Source: CAD feature listing. Evaluate the final solid. Frame: model axes, mm. Face numbers are marked on the shaded views. A direction names the side the tool comes from. Give positions to 0.01 mm unless a question says otherwise; leave off trailing zeros. Write each loop counter-clockwise with the first axis right and the second up, starting at its lowest first coordinate (ties: lowest second). Pieces come first, ordered by that corner, then holes. Notation, with made-up numbers: M 46.25,34.5 L 87.25,34.5 A25 ccw 87.25,58.5 Z; hole C -7.75,-1 d11. An arc over 180 degrees is marked long. Answer as a JSON object with one key per item and string values. Group by question number.
```python
from build123d import *

# Parameters (mm, degrees)
F0_W     = 177.8
F0_H     = 152.4
F1_DEPTH = 81.59288
F2_R     = 63.5
F3_DEPTH = 51.22014
F4_R     = 5.08
F5_R     = 5.08
F6_T     = -2.54


with BuildPart() as f1:
    # F0 (on Front) → F1 (new body)
    with BuildSketch(Plane.XZ):
        Rectangle(F0_W, F0_H)
    extrude(amount=-F1_DEPTH)

    # F2 (on face) → F3 (join)
    with BuildSketch(Plane(origin=(0, 81.59288, 0), x_dir=(-1, 0, 0), z_dir=(0, 1, 0))):
        Circle(F2_R)
    extrude(amount=F3_DEPTH)

    # F4
    f4_edges = [f1.edges().sort_by_distance(p)[0] for p in [
        (63.5, 81.59288, 0),
        (63.5, 132.81302, 0),
        (-88.9, 40.79644, 76.2),
        (88.9, 40.79644, 76.2),
        (-88.9, 40.79644, -76.2),
        (88.9, 40.79644, -76.2),
    ]]
    fillet(f4_edges, radius=F4_R)

    # F5
    f5_edges = [f1.edges().sort_by_distance(p)[0] for p in [
        (0, 81.59288, -76.2),
    ]]
    fillet(f5_edges, radius=F5_R)

    # F6
    f6_openings = [f1.faces().sort_by_distance(p)[0] for p in [
        (0, 0, 0),
    ]]
    offset(amount=F6_T, openings=f6_openings)


solid = f1.part
```
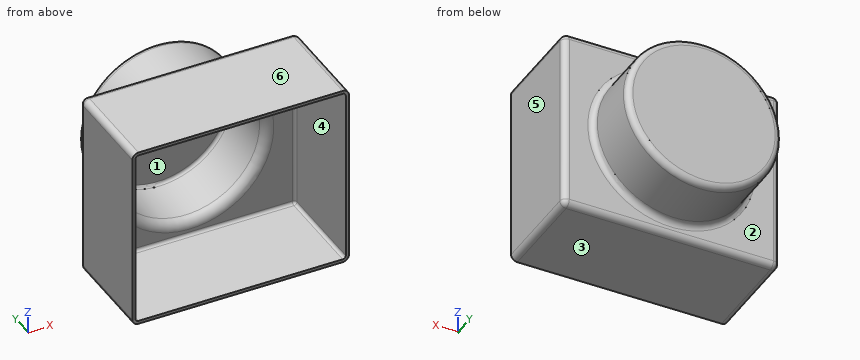
(1) Pull-direction query (Z, two-part tool) for the marked faces 4, 5 and 6; classes: pulls with the +Z half, pulls with the -Z half, needs draft (parallel to the pull), parting line crosses it, or undercut.
(2) Contact query for flat-ended pins moving along their axis: pin 1 Ø6 at (y, z) = (111, 50.5) entering from -X; pin 2 Ø2 at (x, y) = (28, 79.5) entering from +Z; pin 3 Ø6 at (y, z) = (81.5, 29) entering from +X. Output: stop coordinate, or through.
(3) Section A-A, the plane y = 12.5. Return loops of the section in (x, z).
(4) Access query for the marked faces 1, 2 and 3. Directions: +Z, -Z, +X, -X, +Y, -Y. A direction counts if a zero-diameter tool reaches every point of the face in a straight line with its end or side. Return the directions, or none.
(5) Section B-B, the plane x = 0. Return loops of the section in (y, z), plus the area to 3 significant figures.
(6) Section C-C, the plane z = 0. Return loops of the section in (x, y), plus the area to 3 significant figures.
(7) Ray query, L1, parallel to X at y = 63, z = 43.5; L2, parallel to Z at x = 0, y = 117; L3, parallel to X at y = 126, z = -2. Return the intervals inside material, ascending. Write a range as [from, to].
Reported:
{
 "1": {"face 4": "undercut", "face 5": "needs draft", "face 6": "pulls with the +Z half"},
 "2": {"pin 1": "stops at x = -42.14", "pin 2": "stops at z = 75.8", "pin 3": "stops at x = 88.5"},
 "3": {"outline": "M -88.9,-71.12 A5.08 ccw -83.82,-76.2 L 83.82,-76.2 A5.08 ccw 88.9,-71.12 L 88.9,71.12 A5.08 ccw 83.82,76.2 L -83.82,76.2 A5.08 ccw -88.9,71.12 Z; hole M -86.36,-71.12 A2.54 ccw -83.82,-73.66 L 83.82,-73.66 A2.54 ccw 86.36,-71.12 L 86.36,71.12 A2.54 ccw 83.82,73.66 L -83.82,73.66 A2.54 ccw -86.36,71.12 Z"},
 "4": {"face 1": "-Y", "face 2": "+Y", "face 3": "-Z, +X, -X, +Y, -Y"},
 "5": {"outline": "M 0,-76.2 L 76.51,-76.2 A5.08 ccw 81.59,-71.12 L 81.59,-68.58 A5.08 cw 86.67,-63.5 L 127.73,-63.5 A5.08 ccw 132.81,-58.42 L 132.81,58.42 A5.08 ccw 127.73,63.5 L 86.67,63.5 A5.08 cw 81.59,68.58 L 81.59,71.12 A5.08 ccw 76.51,76.2 L 0,76.2 L 0,73.66 L 76.51,73.66 A2.54 cw 79.05,71.12 L 79.05,68.58 A7.62 ccw 86.67,60.96 L 127.73,60.96 A2.54 cw 130.27,58.42 L 130.27,-58.42 A2.54 cw 127.73,-60.96 L 86.67,-60.96 A7.62 ccw 79.05,-68.58 L 79.05,-71.12 A2.54 cw 76.51,-73.66 L 0,-73.66 Z", "area": "1,020 mm2"},
 "6": {"outline": "M -88.9,0 L -86.36,0 L -86.36,76.51 A2.54 cw -83.82,79.05 L -68.58,79.05 A7.62 ccw -60.96,86.67 L -60.96,127.73 A2.54 cw -58.42,130.27 L 58.42,130.27 A2.54 cw 60.96,127.73 L 60.96,86.67 A7.62 ccw 68.58,79.05 L 83.82,79.05 A2.54 cw 86.36,76.51 L 86.36,0 L 88.9,0 L 88.9,76.51 A5.08 ccw 83.82,81.59 L 68.58,81.59 A5.08 cw 63.5,86.67 L 63.5,127.73 A5.08 ccw 58.42,132.81 L -58.42,132.81 A5.08 ccw -63.5,127.73 L -63.5,86.67 A5.08 cw -68.58,81.59 L -83.82,81.59 A5.08 ccw -88.9,76.51 Z", "area": "1,080 mm2"},
 "7": {"L1": "x = [-88.9, -86.36], [86.36, 88.9]", "L2": "z = [-63.5, -60.96], [60.96, 63.5]", "L3": "x = [-63.47, -60.93], [60.93, 63.47]"}
}
